Autodesk Inventor part; units mm, degrees
ref_plane "YZ Plane" through (0, 0, 0) normal (1, 0, 0) x (0, 1, 0)
ref_plane "XZ Plane" through (0, 0, 0) normal (0, 1, 0) x (-1, 0, 0)
ref_plane "XY Plane" through (0, 0, 0) normal (0, 0, 1) x (1, 0, 0)
sketch "Sketch1" plane through (0, 0, 0) normal (0, 0, 1) x (1, 0, 0)
  circle A0 centre (0, 0) radius 3
  dimension "d0" = 6
extrude "Extrusion1" add sketch "Sketch1" along normal blind 35
sketch "Sketch2" plane through (0, 0, 0) normal (0, 0, -1) x (-1, 0, 0)
  circle A0 centre (0, 0) radius 3
  circle A1 centre (0, 0) radius 5
  dimension "d3" = 10
extrude "Extrusion2" add sketch "Sketch2" along normal blind 6 contours A0 | A1
sketch "Sketch3" plane through (0, 0, -6) normal (0, 0, -1) x (-1, 0, 0)
  circle A0 centre (0, 0) radius 5
  line L0 (-1.4434, 2.5) -> (1.4434, 2.5)
  line L1 (1.4434, 2.5) -> (2.8868, 0)
  line L2 (2.8868, 0) -> (1.4434, -2.5)
  line L3 (1.4434, -2.5) -> (-1.4434, -2.5)
  line L4 (-1.4434, -2.5) -> (-2.8868, 0)
  line L5 (-2.8868, 0) -> (-1.4434, 2.5)
  dimension "d6" = 5
extrude "Extrusion3" cut sketch "Sketch3" against normal blind 3 contours L0 L1 L2 L3 L4 L5
thread "Thread1"
chamfer "Chamfer1" distance 0.508 angle 45 3 edges at (5, 0, -6) (5, 0, 0) (-3, 0, 35)
properties part number "M6 x 12mm" material "Steel"
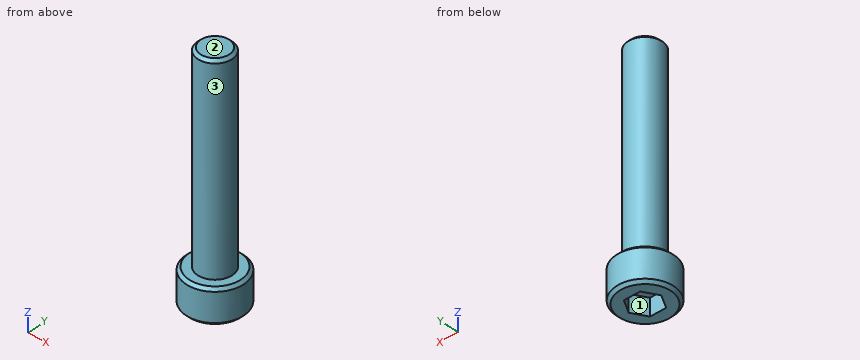
The model under review builds one solid part; all positions refer to its coordinate system, in mm. Face numbers are marked on the shaded views. Give positions to 0.01 mm unless a question says otherwise; leave off trailing zeros. Order: outer loops, then holes, each group sorted by start corner. A loop starts at its lowest first (then second) coordinate and runs counter-clockwise, first axis right, second up. Notation, with made-up numbers: M 4.25,55.5 L 43.25,55.5 A18 cw 43.25,79.5 Z; hole C 60.5,26 d4. An arc over 180 degrees is marked long. Use one line per item in the form item = value. Start each with the question number.
Item 1: Insertion check: pin 1 Ø1.5 at (x, y) = (-3.5, 4) entering from -Z; pin 2 Ø3 at (y, z) = (3.5, 30) entering from +X; pin 3 Ø1 at (y, z) = (-0.5, 12.5) entering from +X. Each pin has a flat end and moves straight along its axis. Give the tip position at first contact, or say it passes through.
Item 2: To check wall thickness, follow line 1 along Z through (x, y) = (1, 2); line 2 along Y through (x, z) = (0, 11.5); line 3 along Z through (x, y) = (0.25, 4). State the ranges of each line that lie inside material, in increasing order. Write a range as from..to.
Item 3: We need section A-A on x = 0. Give the boundary of the cut face in (y, z).
Item 4: We need section B-B on z = 1.5. Give the boundary of the cut face in (x, y).
Item 5: The part is to be moulded in two halves that separate along Y. For the marked faces 1, 2 and 3, say which applies: pulls with the +Y half, pulls with the -Y half, needs draft (parallel to the pull), parting line crosses it, or undercut.
Completed:
q1.pin_1 = -5.93
q1.pin_2 = 2.24
q1.pin_3 = 3
q2.line_1 = -3..35
q2.line_2 = -3..3
q2.line_3 = -6..0
q3.outline = M -5,-5.49 L -4.49,-6 L -2.5,-6 L -2.5,-3 L 2.5,-3 L 2.5,-6 L 4.49,-6 L 5,-5.49 L 5,-0.51 L 4.49,0 L 3,0 L 3,34.49 L 2.49,35 L -2.49,35 L -3,34.49 L -3,0 L -4.49,0 L -5,-0.51 Z
q4.outline = C 0,0 d6
q5.face_1 = undercut
q5.face_2 = needs draft
q5.face_3 = parting line crosses it
